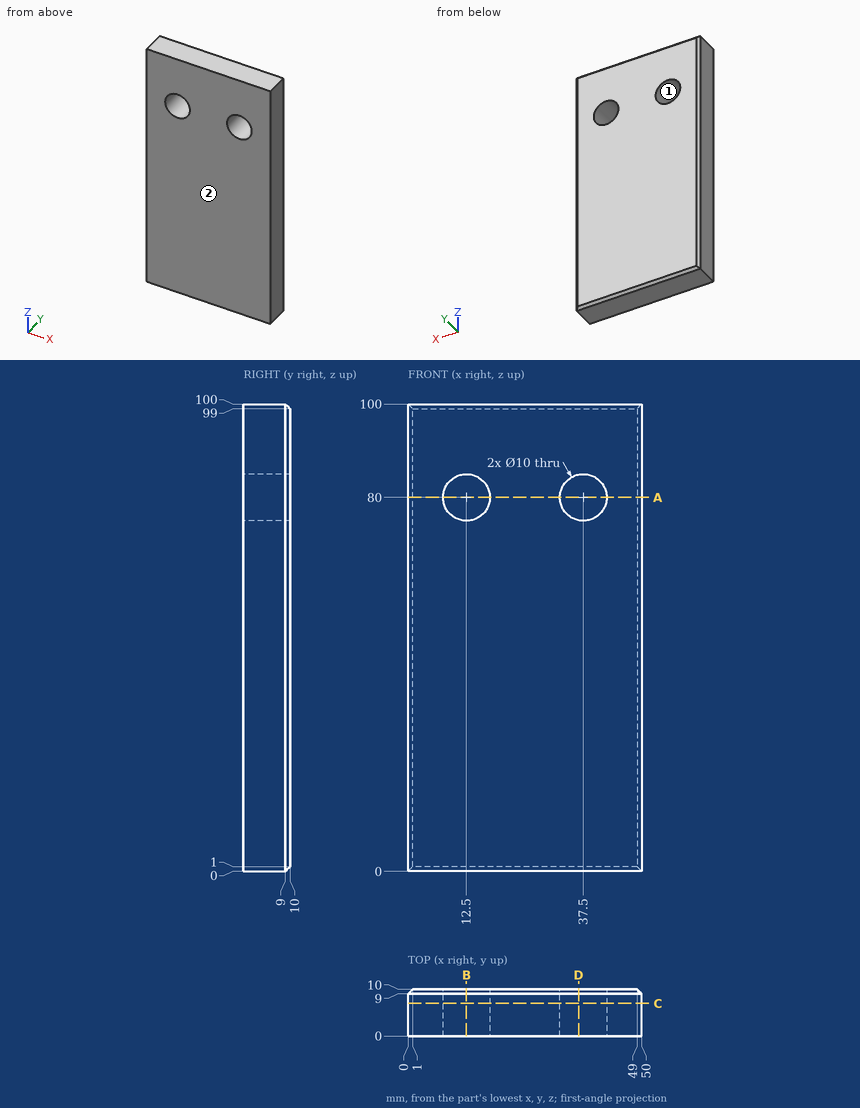
Answer from the drawing. Dimensions are ordinates in mm from the lowest x, y and z of the part. Coordinates: 2 decimals unless noted, no trailing zeros. Loops run counter-clockwise (first coordinate to the right, second up) from the corner with the lowest first, then second, coordinate; pieces in that order, holes last. Notation, with made-up numbers: (11, 3) -> (54, 3) arc R13 ccw to (54, 10) -> close; hole circle Ø7 at (45.25, 28.5). An arc over 180 degrees is marked (long way). Return JSON: item names as keys, results as strings.
Item 1: Find section B-B (x = 12.5). Determine the outline of the cut face in (y, z).
Answers:
{"outline": "(0, 0) -> (9, 0) -> (10, 1) -> (10, 75) -> (0, 75) -> close; (0, 85) -> (10, 85) -> (10, 99) -> (9, 100) -> (0, 100) -> close"}
Item 2: A flat-ended cylindrical pin translates along its axis: P1, Ø8, axis at x = 37.5, z = 80, coming from the +Y side. Find the tip coordinate at first contact, or state that the pin passes through.
Answers:
{"P1": "passes through"}
Item 3: Find section C-C (y = 7). Determine the outline of the cut face in (x, z), plus the area to 3 significant figures.
Answers:
{"outline": "(0, 0) -> (50, 0) -> (50, 100) -> (0, 100) -> close; hole circle Ø10 at (12.5, 80); hole circle Ø10 at (37.5, 80)", "area": "4,840 mm2"}
Item 4: Find the intervals of material crossed by probe 1 along Z at (x, y) = (12.5, 5.25); probe 2 along X at (y, z) = (7.25, 81); probe 3 along X at (y, z) = (3.75, 75.5), in increasing order.
Answers:
{"probe 1": "z = 0 to 75, 85 to 100", "probe 2": "x = 0 to 7.6, 17.4 to 32.6, 42.4 to 50", "probe 3": "x = 0 to 10.32, 14.68 to 35.32, 39.68 to 50"}
Item 5: Find section A-A (z = 80). Determine the outline of the cut face in (x, y), plus the area to 3 significant figures.
Answers:
{"outline": "(0, 0) -> (7.5, 0) -> (7.5, 10) -> (1, 10) -> (0, 9) -> close; (17.5, 0) -> (32.5, 0) -> (32.5, 10) -> (17.5, 10) -> close; (42.5, 0) -> (50, 0) -> (50, 9) -> (49, 10) -> (42.5, 10) -> close", "area": "299 mm2"}
Item 6: For a pull along X with two mould halves and no side action, classify the marked faces 1 and 2 as +X half, -X half, draft (parallel to the pull), parting line (faces both ways), or undercut.
Answers:
{"face 1": "undercut", "face 2": "draft"}
Item 7: Find section D-D (x = 36.5). Determine the outline of the cut face in (y, z).
Answers:
{"outline": "(0, 0) -> (9, 0) -> (10, 1) -> (10, 75.1) -> (0, 75.1) -> close; (0, 84.9) -> (10, 84.9) -> (10, 99) -> (9, 100) -> (0, 100) -> close"}
